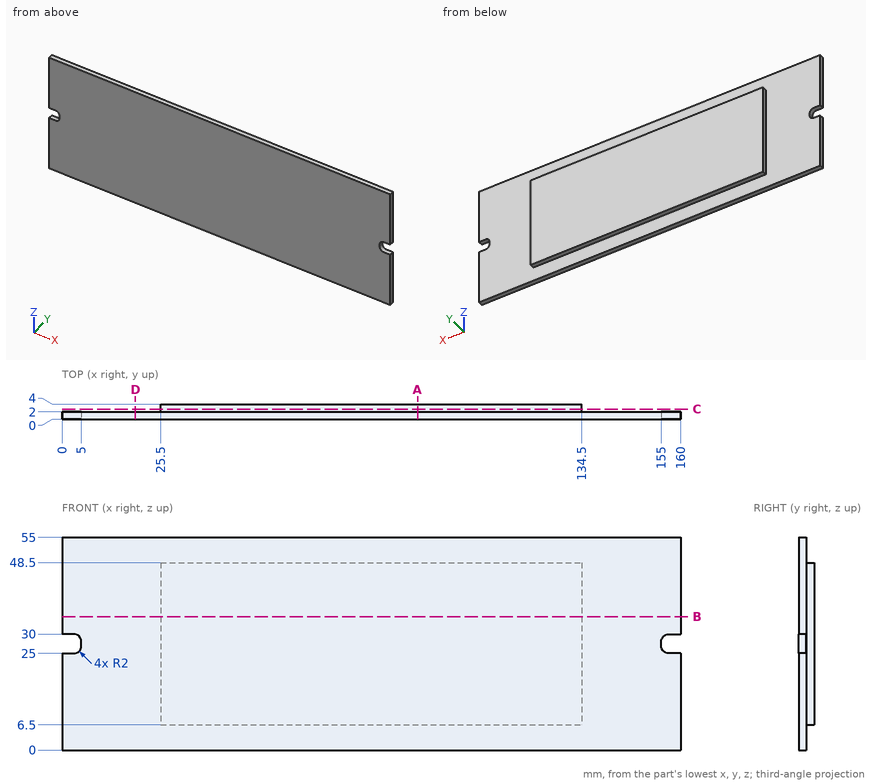
Drawing for the job (mm, zero at the part's lowest x, y, z). Round coordinates to 2 decimals unless told otherwise and drop trailing zeros. Write each loop counter-clockwise with the first axis right and the second up, starting at its lowest first coordinate (ties: lowest second). Pieces come first, ordered by that corner, then holes.
Item 1: Band-saw the part on B-B on z = 34.5. Write the cut outline in (x, y), then the cut area to 3 significant figures.
Filled in:
outline: (0, 0) - (160, 0) - (160, 2) - (134.5, 2) - (134.5, 4) - (25.5, 4) - (25.5, 2) - (0, 2) - close
area: 538 mm2
Item 2: Band-saw the part on C-C on y = 2.7. Write the cut outline in (x, z), then the cut area to 3 significant figures.
Filled in:
outline: (25.5, 6.5) - (134.5, 6.5) - (134.5, 48.5) - (25.5, 48.5) - close
area: 4,580 mm2
Item 3: Band-saw the part on D-D on x = 19. Write the cut outline in (y, z), then the cut area to 3 significant figures.
Filled in:
outline: (0, 0) - (2, 0) - (2, 55) - (0, 55) - close
area: 110 mm2
Item 4: Band-saw the part on A-A on x = 92. Write the cut outline in (y, z).
Filled in:
outline: (0, 0) - (2, 0) - (2, 6.5) - (4, 6.5) - (4, 48.5) - (2, 48.5) - (2, 55) - (0, 55) - close
Item 5: Drill centre lines: L1, parallel to X at y = 3.75, z = 42.5; L2, parallel to Y at x = 138.5, z = 39.5; L3, parallel to Z at x = 81.5, y = 3.15. Where is each one in solid material? Low to high.
Filled in:
L1: x = 25.5 to 134.5
L2: y = 0 to 2
L3: z = 6.5 to 48.5
Item 6: Drop flat-ended pins along their axis: pin 1 Ø1.6 at (y, z) = (3, 22.5) entering from -X; pin 2 Ø0.5 at (y, z) = (1, 27.5) entering from -X; pin 3 Ø1.1 at (y, z) = (0.5, 27.5) entering from +X. Give the stop position or say it passes through.
Filled in:
pin 1: stops at x = 25.5
pin 2: stops at x = 5
pin 3: stops at x = 155
